```python
from build123d import *

# Parameters (mm, degrees)
F0_W      = 203.2
F0_H      = 203.2
F1_DEPTH  = 1.6002
F2_R      = 31.75
F2_R_2    = 2.2479
F3_DEPTH  = 1.6002
F5_DEPTH  = 9.525
F7_DEPTH  = 1.6002
F9_W      = 203.2
F9_H      = 203.2
F9_W_2    = 200.152
F9_H_2    = 200.152
F10_DEPTH = 65.024
F11_W     = 203.2
F11_H     = 203.2
F11_R     = 58.42
F12_DEPTH = 1.524
F13_R     = 59.944
F13_R_2   = 58.42
F14_DEPTH = 16.51


with BuildPart() as f1:
    # F0 (on Top) → F1 (new body)
    with BuildSketch(Plane.XY):
        Rectangle(F0_W, F0_H)
    extrude(amount=-F1_DEPTH)

    # F2 (on face) → F3 (cut, through all)
    with BuildSketch(Plane.XY):
        Circle(F2_R)
        with Locations((0, 39.37)):
            Circle(F2_R_2)
        with Locations((-39.37, 0)):
            Circle(F2_R_2)
        with Locations((0, -39.37)):
            Circle(F2_R_2)
        with Locations((39.37, 0)):
            Circle(F2_R_2)
    extrude(amount=-F3_DEPTH, mode=Mode.SUBTRACT)

    # F4 (on Front) → F5 (join, symmetric)
    with BuildSketch(Plane.XZ):
        Polygon((57.15, -1.6002), (44.45, -1.6002), (44.45, -3.2004), (55.5498, -3.2004), (55.5498, -65.1002), (57.15, -65.1002), align=None)
        Polygon((-57.15, -1.6002), (-57.15, -65.1002), (-55.5498, -65.1002), (-55.5498, -3.2004), (-44.45, -3.2004), (-44.45, -1.6002), align=None)
    extrude(amount=F5_DEPTH, both=True)

    # F6 (on face) → F7 (join)
    with BuildSketch(Plane(origin=(0, 0, -65.1002), x_dir=(1, 0, 0), z_dir=(0, 0, -1))):
        Polygon((47.9298, -9.525), (57.15, -9.525), (57.15, 9.525), (47.9298, 9.525), (47.9298, 4.445), (51.7398, 4.445), (51.7398, 6.0452), (49.53, 6.0452), (49.53, 7.9248), (53.9496, 7.9248), (53.9496, 0), (53.9496, -7.9248), (49.53, -7.9248), (49.53, -6.0452), (51.7398, -6.0452), (51.7398, -4.445), (47.9298, -4.445), align=None)
    extrude(amount=F7_DEPTH)

    # F8: F1 across plane


with BuildPart() as f1_1:
    add(f1.part)
    add(f1.part.mirror(Plane.YZ))

    # F9 (on face) → F10 (join)
    with BuildSketch(Plane(origin=(0, 0, -1.6002), x_dir=(1, 0, 0), z_dir=(0, 0, -1))):
        Rectangle(F9_W, F9_H)
        Rectangle(F9_W_2, F9_H_2, mode=Mode.SUBTRACT)
    extrude(amount=F10_DEPTH)

    # F11 (on face) → F12 (join)
    with BuildSketch(Plane(origin=(0, 0, -66.6242), x_dir=(1, 0, 0), z_dir=(0, 0, -1))):
        Rectangle(F11_W, F11_H)
        Circle(F11_R, mode=Mode.SUBTRACT)
    extrude(amount=F12_DEPTH)

    # F13 (on face) → F14 (join)
    with BuildSketch(Plane(origin=(0, 0, -68.1482), x_dir=(1, 0, 0), z_dir=(0, 0, -1))):
        Circle(F13_R)
        Circle(F13_R_2, mode=Mode.SUBTRACT)
    extrude(amount=F14_DEPTH)


solid = f1_1.part
```
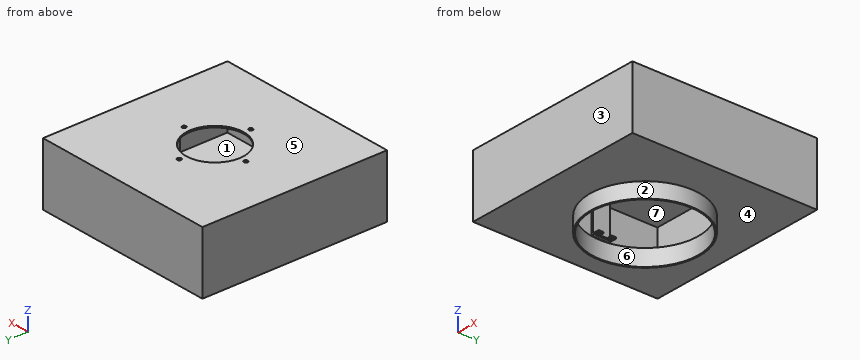
Check sheet for the modelled part. Datum: model origin and axes. Units: mm. Face numbers are marked on the shaded views. A direction names the side the tool comes from. Coordinates: 2 decimals unless noted, no trailing zeros. Loops run counter-clockwise (first coordinate to the right, second up) from the corner with the lowest first, then second, coordinate; pieces in that order, holes last.
1) Sectioned sample at A-A (z = -12.5). Record the boundary of the cut face in (x, y) (3 decimals).
2) Release check for a two-part mould opening along Y. For the marked faces 1, 2, 3 and 4 record: released by +Y, released by -Y, zero draft, split by the parting line, or undercut.
3) Access from +Z, -Z, +X, -X, +Y, -Y to the whole of each face (thin tool, end or side, straight path). Record for the marked faces 5, 6 and 7.
4) Sectioned sample at B-B (y = 78). Record the boundary of the cut face in (x, z).
5) Sectioned sample at D-D (x = -21). Record the boundary of the cut face in (y, z), and give its area (3 significant figures).
6) Material ranges on probe 1 along X at (y, z) = (82.5, -8); probe 2 along Z at (x, y) = (-29.5, -86.5), recorded low to high.
7) Gauge pin test, flat ends, axial feed: pin 1 (2 mm diameter, centred on x = -25, y = 39, fed in from -Z); pin 2 (1 mm diameter, centred on x = -24, y = 62.5, fed in from -Z); pin 3 (7.5 mm diameter, centred on x = -54.5, y = 1.5, fed in from -Z). Record the tip position at first contact, or that the pin passes through.
Check sheet entries:
1. outline: (-101.6, -101.6) - (101.6, -101.6) - (101.6, 101.6) - (-101.6, 101.6) - close; (-57.15, -9.525) - (-55.55, -9.525) - (-55.55, 9.525) - (-57.15, 9.525) - close; (55.55, -9.525) - (57.15, -9.525) - (57.15, 9.525) - (55.55, 9.525) - close; hole (-100.076, -100.076) - (100.076, -100.076) - (100.076, 100.076) - (-100.076, 100.076) - close
2. face 1: undercut
2. face 2: split by the parting line
2. face 3: released by -Y
2. face 4: zero draft
3. face 5: +Z, +X, -X, +Y, -Y
3. face 6: -Z
3. face 7: none
4. outline: (-101.6, -68.15) - (101.6, -68.15) - (101.6, 0) - (-101.6, 0) - close; hole (-100.08, -66.62) - (100.08, -66.62) - (100.08, -1.6) - (-100.08, -1.6) - close
5. outline: (-101.6, -68.15) - (-56.15, -68.15) - (-56.15, -84.66) - (-54.52, -84.66) - (-54.52, -66.62) - (-100.08, -66.62) - (-100.08, -1.6) - (-23.81, -1.6) - (-23.81, 0) - (-101.6, 0) - close; (23.81, -1.6) - (100.08, -1.6) - (100.08, -66.62) - (54.52, -66.62) - (54.52, -84.66) - (56.15, -84.66) - (56.15, -68.15) - (101.6, -68.15) - (101.6, 0) - (23.81, 0) - close
5. area: 644 mm2
6. probe 1: x = -101.6 to -100.08, 100.08 to 101.6
6. probe 2: z = -68.15 to -66.62, -1.6 to 0
7. pin 1: stops at z = -1.6
7. pin 2: stops at z = -68.15
7. pin 3: stops at z = -66.7
